```python
from build123d import *

# Parameters (mm, degrees)
F0_R      = 9
F0_R_2    = 6.1
F1_DEPTH  = 4
F2_R      = 8
F2_R_2    = 6.1
F3_DEPTH  = 2
F4_R      = 9
F4_R_2    = 8
F4_R_3    = 6.1
F5_DEPTH  = 4
F6_R      = 8
F6_R_2    = 6.1
F7_DEPTH  = 2
F8_R      = 9
F8_R_2    = 8
F8_R_3    = 6.1
F9_DEPTH  = 50
F10_R     = 8
F10_R_2   = 6.1
F11_DEPTH = 2
F12_R     = 6.1
F13_DEPTH = 3


with BuildPart() as f1:
    # F0 (on Top) → F1 (new body)
    with BuildSketch(Plane.XY):
        Circle(F0_R)
        Circle(F0_R_2, mode=Mode.SUBTRACT)
    extrude(amount=F1_DEPTH)

    # F2 (on face) → F3 (join)
    with BuildSketch(Plane.XY.offset(4)):
        Circle(F2_R)
        Circle(F2_R_2, mode=Mode.SUBTRACT)
    extrude(amount=F3_DEPTH)

    # F4 (on face) → F5 (join)
    with BuildSketch(Plane.XY.offset(6)):
        Circle(F4_R)
        Circle(F4_R_2, mode=Mode.SUBTRACT)
        Circle(F4_R_2)
        Circle(F4_R_3, mode=Mode.SUBTRACT)
    extrude(amount=F5_DEPTH)

    # F6 (on face) → F7 (join)
    with BuildSketch(Plane.XY.offset(10)):
        Circle(F6_R)
        Circle(F6_R_2, mode=Mode.SUBTRACT)
    extrude(amount=F7_DEPTH)

    # F8 (on face) → F9 (join)
    with BuildSketch(Plane.XY.offset(12)):
        Circle(F8_R)
        Circle(F8_R_2, mode=Mode.SUBTRACT)
        Circle(F8_R_2)
        Circle(F8_R_3, mode=Mode.SUBTRACT)
    extrude(amount=F9_DEPTH)

    # F10 (on face) → F11 (join)
    with BuildSketch(Plane.XY.offset(62)):
        Circle(F10_R)
        Circle(F10_R_2, mode=Mode.SUBTRACT)
    extrude(amount=F11_DEPTH)

    # F12 (on face) → F13 (join)
    with BuildSketch(Plane.XY.offset(64)):
        with BuildLine():
            ThreePointArc((8, 0), (5.6568542495, 5.6568542495), (0, 8))
            ThreePointArc((0, 8), (-5.6568542495, 5.6568542495), (-8, 0))
            ThreePointArc((-8, 0), (-5.6568542495, -5.6568542495), (0, -8))
            ThreePointArc((0, -8), (5.6568542495, -5.6568542495), (8, 0))
        make_face()
        Circle(F12_R, mode=Mode.SUBTRACT)
        with BuildLine():
            Line((0, 8), (-8, 8))
            Line((-8, 8), (-8, 0))
            ThreePointArc((-8, 0), (-5.6568542495, 5.6568542495), (0, 8))
        make_face()
        with BuildLine():
            ThreePointArc((0, -8), (-5.6568542495, -5.6568542495), (-8, 0))
            Line((-8, 0), (-8, -8))
            Line((-8, -8), (0, -8))
        make_face()
        with BuildLine():
            Line((8, -8), (8, 0))
            ThreePointArc((8, 0), (5.6568542495, -5.6568542495), (0, -8))
            Line((0, -8), (8, -8))
        make_face()
        with BuildLine():
            Line((8, 8), (0, 8))
            ThreePointArc((0, 8), (5.6568542495, 5.6568542495), (8, 0))
            Line((8, 0), (8, 8))
        make_face()
    extrude(amount=F13_DEPTH)


solid = f1.part
```
Can you work these out from the model? Positions are in its coordinate system, mm. A direction names the side the tool comes from. Give positions to 0.01 mm unless a question says otherwise; leave off trailing zeros. Order: outer loops, then holes, each group sorted by start corner. A loop starts at its lowest first (then second) coordinate and runs counter-clockwise, first axis right, second up. Notation, with made-up numbers: M -1.75,13.25 L 56.25,13.25 A15 cw 56.25,39.25 Z; hole C -34,85 d5. An arc over 180 degrees is marked long. Write item = value, one per line. Start each with the question number.
Q1. We'd pull the mould along Z, two halves only. Please class faces 4 (the flat face through (8, 0, 65)), 5 (the flat face through (3.4, 5.4, 67)), 6 (the flat face through (6, 6, 64)): pulls with the +Z half, pulls with the -Z half, needs draft (parallel to the pull), parting line crosses it, or undercut.
Q2. Suppose I cut it at C-C (z = 58). Write out the boundary of the cut face in (x, y).
Q3. For faces 1 (the cylindrical face through (-1.73, -7.81, 10.99)), 2 (the flat face through (-6, 6, 64)), 3 (the flat face through (6, -6, 64)), which set-ups out of +Z, -Z, +X, -X, +Y, -Y let a thin tool reach every point of the face, with its end or its side?
Q4. Will these pins go through, and if not, where does the flat tip stop? pin 1 Ø2 at (x, z) = (2, 26.5) entering from -Y; pin 2 Ø2.5 at (x, z) = (-2, 66) entering from -Y; pin 3 Ø4 at (x, y) = (-5.5, -4) entering from -Z; pin 4 Ø1.5 at (y, z) = (-2.5, 65) entering from -X.
Q5. I need wall thicknesses on probe 1 along Z at (x, y) = (3.25, -7.5); probe 2 along Z at (x, y) = (8.5, -1.5); probe 3 along Y at (x, z) = (0, 52.5). Which ranges of each line are inside material? Lowest first, please. Write a range as [from, to].
Q6. Suppose I cut it at D-D (y = -6.75). Write out the boundary of the cut face in (x, z).
Check result:
q1.face_4 = needs draft
q1.face_5 = pulls with the +Z half
q1.face_6 = undercut
q2.outline = C 0,0 d18; hole C 0,0 d12.2
q3.face_1 = none
q3.face_2 = -X, +Y
q3.face_3 = +X, -Y
q4.pin_1 = -8.94
q4.pin_2 = -8
q4.pin_3 = 0
q4.pin_4 = -8
q5.probe_1 = [0, 4], [6, 10], [12, 62], [64, 67]
q5.probe_2 = [0, 4], [6, 10], [12, 62]
q5.probe_3 = [-9, -6.1], [6.1, 9]
q6.outline = M -8,64 L -4.29,64 L -4.29,62 L -5.95,62 L -5.95,12 L -4.29,12 L -4.29,10 L -5.95,10 L -5.95,6 L -4.29,6 L -4.29,4 L -5.95,4 L -5.95,0 L 5.95,0 L 5.95,4 L 4.29,4 L 4.29,6 L 5.95,6 L 5.95,10 L 4.29,10 L 4.29,12 L 5.95,12 L 5.95,62 L 4.29,62 L 4.29,64 L 8,64 L 8,67 L -8,67 Z
